The listing builds one solid part. Answer for the finished solid, in the listing's coordinates (mm). Give positions to 0.01 mm unless a question says otherwise; leave off trailing zeros. Order: outer loops, then holes, each group sorted by start corner. A loop starts at its lowest first (then second) coordinate and runs counter-clockwise, first axis right, second up. Notation, with made-up numbers: M 46,53 L 71,53 A5 cw 71,59 Z; hole C 48,75.25 d7. An arc over 180 degrees is marked long. Answer as a JSON object with one key per item and string values. Group by question number.
```python
from build123d import *

# Parameters (mm, degrees)
PEG_DEPTH      = 2.5
TAIL_BASE_W    = 0.64
TAIL_BASE_H    = 0.64
TAIL_DEPTH     = 3.05
HEAD_BASE_W    = 0.64
HEAD_BASE_H    = 0.64
HEAD_DEPTH     = 5.84
MULTIPLY_COUNT = 2
MULTIPLY_PITCH = 2.54


with BuildPart() as part:
    # peg base → peg (new body)
    with BuildSketch(Plane.XY):
        Polygon((0.845735931, -1.27), (1.27, -0.845735931), (1.27, 0.845735931), (0.845735931, 1.27), (-0.845735931, 1.27), (-1.27, 0.845735931), (-1.27, -0.845735931), (-0.845735931, -1.27), align=None)
    peg = extrude(amount=PEG_DEPTH)

    # tail base → tail (add)
    with BuildSketch(Plane(origin=(0, 0, 0), x_dir=(-1, 0, 0), z_dir=(0, 0, -1))):
        Rectangle(TAIL_BASE_W, TAIL_BASE_H)
    tail = extrude(amount=TAIL_DEPTH)

    # head base → head (add)
    with BuildSketch(Plane.XY.offset(2.5)):
        Rectangle(HEAD_BASE_W, HEAD_BASE_H)
    head = extrude(amount=HEAD_DEPTH)

    # multiply: peg, tail, head ×2
    with Locations(*[(i * MULTIPLY_PITCH, 0, 0) for i in range(1, MULTIPLY_COUNT)]):
        add(peg)
        add(tail)
        add(head)


solid = part.part
```
Item 1: Flat-ended cylindrical pins translate along their axes: P1, Ø1, axis at y = 0, z = 3.5, coming from the +X side; P2, Ø0.7, axis at x = 2.5, z = -1, coming from the -Y side; P3, Ø0.5, axis at y = 0, z = -1, coming from the -X side. Find the tip coordinate at first contact, or state that the pin passes through.
Item 2: Consider probe 1 along X at (y, z) = (0, -2); probe 2 along Z at (x, y) = (-0.45, 0.8); probe 3 along X at (y, z) = (1.1, 1.75). Determine where each line is inside the solid, lowest interval first. Write a range as from..to.
Item 3: Section B-B (y = 0.2) is taken. Determine the outline of the cut face in (x, z).
Item 4: Section D-D (z = 2) is taken. Determine the outline of the cut face in (x, y), and give its area (3 significant figures).
Item 5: Section A-A (z = -2) is taken. Determine the outline of the cut face in (x, y), and give its area (3 significant figures).
Item 6: Determine the mould class of faces 1 (the flat face through (1, 0, 0)), 2 (the flat face through (3.81, 0, 1)), 3 (the flat face through (3, 1.27, 1)) for opening direction X: released by +X, released by -X, zero draft, split by the parting line, or undercut.
Item 7: Section C-C (x = 2.65) is taken. Determine the outline of the cut face in (y, z), and give its area (3 significant figures).
Values found:
{
 "1": {"P1": "stops at x = 2.86", "P2": "stops at y = -0.32", "P3": "stops at x = -0.32"},
 "2": {"probe 1": "x = -0.32..0.32, 2.22..2.86", "probe 2": "z = 0..2.5", "probe 3": "x = -1.02..1.02, 1.52..3.56"},
 "3": {"outline": "M -1.27,0 L -0.32,0 L -0.32,-3.05 L 0.32,-3.05 L 0.32,0 L 2.22,0 L 2.22,-3.05 L 2.86,-3.05 L 2.86,0 L 3.81,0 L 3.81,2.5 L 2.86,2.5 L 2.86,8.34 L 2.22,8.34 L 2.22,2.5 L 0.32,2.5 L 0.32,8.34 L -0.32,8.34 L -0.32,2.5 L -1.27,2.5 Z"},
 "4": {"outline": "M -1.27,-0.85 L -0.85,-1.27 L 0.85,-1.27 L 1.27,-0.85 L 1.69,-1.27 L 3.39,-1.27 L 3.81,-0.85 L 3.81,0.85 L 3.39,1.27 L 1.69,1.27 L 1.27,0.85 L 0.85,1.27 L -0.85,1.27 L -1.27,0.85 Z", "area": "12.2 mm^2"},
 "5": {"outline": "M -0.32,-0.32 L 0.32,-0.32 L 0.32,0.32 L -0.32,0.32 Z; M 2.22,-0.32 L 2.86,-0.32 L 2.86,0.32 L 2.22,0.32 Z", "area": "0.819 mm^2"},
 "6": {"face 1": "undercut", "face 2": "released by +X", "face 3": "zero draft"},
 "7": {"outline": "M -1.27,0 L -0.32,0 L -0.32,-3.05 L 0.32,-3.05 L 0.32,0 L 1.27,0 L 1.27,2.5 L 0.32,2.5 L 0.32,8.34 L -0.32,8.34 L -0.32,2.5 L -1.27,2.5 Z", "area": "12.0 mm^2"}
}
